```python
from build123d import *

# Parameters (mm, degrees)
BOSS_EXTRUDE1_DEPTH = 80
SKETCH2_R           = 21.75
CUT_EXTRUDE1_DEPTH  = 10
SKETCH3_R           = 1.4
CUT_EXTRUDE2_DEPTH  = 4
CUT_EXTRUDE3_DEPTH  = 6
SKETCH5_R           = 2.25
CUT_EXTRUDE4_DEPTH  = 81
SKETCH6_W           = 10.75
SKETCH6_H           = 28.5
CUT_EXTRUDE5_DEPTH  = 28.5
BOSS_EXTRUDE2_DEPTH = 100
SKETCH8_W           = 5
SKETCH8_H           = 28.5
CUT_EXTRUDE6_DEPTH  = 80
SKETCH9_R           = 24
CUT_EXTRUDE7_DEPTH  = 80
SKETCH12_R          = 6
CUT_EXTRUDE9_DEPTH  = 28
SKETCH13_W          = 58.5
SKETCH13_H          = 5
CUT_EXTRUDE10_DEPTH = 28.5
FILLET2_R           = 2
SKETCH15_R          = 1.5
CUT_EXTRUDE11_DEPTH = 28.5


with BuildPart() as part:
    # Sketch1 → Boss-Extrude1 (new body)
    with BuildSketch(Plane(origin=(0, 0, 0), x_dir=(1, 0, 0), z_dir=(0, 1, 0))):
        Polygon((-40, -13.75), (40, -13.75), (40, 13.75), (29.25, 13.75), (29.25, -3.75), (-29.25, -3.75), (-29.25, 13.75), (-40, 13.75), align=None)
    extrude(amount=BOSS_EXTRUDE1_DEPTH)

    # Sketch2 → Cut-Extrude1 (cut)
    with BuildSketch(Plane.XY.offset(13.75)):
        with Locations((0, 35.5)):
            Circle(SKETCH2_R)
    extrude(amount=-CUT_EXTRUDE1_DEPTH, mode=Mode.SUBTRACT)

    # Sketch3 → Cut-Extrude2 (cut)
    with BuildSketch(Plane.XY.offset(13.75)):
        with Locations((26, 65)):
            Circle(SKETCH3_R)
        with Locations((-26, 65)):
            Circle(SKETCH3_R)
    extrude(amount=-CUT_EXTRUDE2_DEPTH, mode=Mode.SUBTRACT)

    # Sketch4 → Cut-Extrude3 (cut)
    with BuildSketch(Plane(origin=(0, 0, 3.75), x_dir=(-1, 0, 0), z_dir=(0, 0, -1))):
        Polygon((-27.21, 62.904218523), (-28.42, 65), (-27.21, 67.095781477), (-24.79, 67.095781477), (-23.58, 65), (-24.79, 62.904218523), align=None)
        Polygon((28.42, 65), (27.21, 67.095781477), (24.79, 67.095781477), (23.58, 65), (24.79, 62.904218523), (27.21, 62.904218523), align=None)
    extrude(amount=-CUT_EXTRUDE3_DEPTH, mode=Mode.SUBTRACT)

    # Sketch5 → Cut-Extrude4 (cut, through all)
    with BuildSketch(Plane(origin=(40, 0, 0), x_dir=(0, 0, -1), z_dir=(1, 0, 0))):
        with Locations((5.75, 18.5)):
            Circle(SKETCH5_R)
        with Locations((5.75, 37)):
            Circle(SKETCH5_R)
    extrude(amount=-CUT_EXTRUDE4_DEPTH, mode=Mode.SUBTRACT)

    # Sketch6 → Cut-Extrude5 (cut, through all)
    with BuildSketch(Plane.XY.offset(13.75)):
        with Locations((-34.625, 65.75)):
            Rectangle(SKETCH6_W, SKETCH6_H)
        with Locations((34.625, 65.75)):
            Rectangle(SKETCH6_W, SKETCH6_H)
    extrude(amount=-CUT_EXTRUDE5_DEPTH, mode=Mode.SUBTRACT)

    # Sketch7 → Boss-Extrude2 (add)
    with BuildSketch(Plane.ZY.offset(40)):
        Polygon((3.75, 0), (3.75, -22), (13.75, -22), (13.75, 0), (13.75, 80), (3.75, 80), align=None)
    extrude(amount=BOSS_EXTRUDE2_DEPTH)

    # Sketch8 → Cut-Extrude6 (cut)
    with BuildSketch(Plane.XY.offset(13.75)):
        with Locations((-42.5, 65.75)):
            Rectangle(SKETCH8_W, SKETCH8_H)
        with Locations((-137.5, 65.75)):
            Rectangle(SKETCH8_W, SKETCH8_H)
    extrude(amount=-CUT_EXTRUDE6_DEPTH, mode=Mode.SUBTRACT)

    # Sketch9 → Cut-Extrude7 (cut)
    with BuildSketch(Plane.XY.offset(13.75)):
        with Locations((-108, 7.5)):
            Circle(SKETCH9_R)
    extrude(amount=-CUT_EXTRUDE7_DEPTH, mode=Mode.SUBTRACT)

    # Sketch12 → Cut-Extrude9 (cut)
    with BuildSketch(Plane.XY.offset(13.75)):
        with Locations((-70, 52)):
            Circle(SKETCH12_R)
    extrude(amount=-CUT_EXTRUDE9_DEPTH, mode=Mode.SUBTRACT)

    # Sketch13 → Cut-Extrude10 (cut, through all)
    with BuildSketch(Plane.XY.offset(13.75)):
        with Locations((0, 77.5)):
            Rectangle(SKETCH13_W, SKETCH13_H)
    extrude(amount=-CUT_EXTRUDE10_DEPTH, mode=Mode.SUBTRACT)

    # Fillet2
    fillet2_edges = [part.edges().sort_by_distance(p)[0] for p in [
        (-29.25, 51.5, 8.75),
        (29.25, 51.5, 8.75),
        (40, 51.5, 0),
        (-40, 0, 8.75),
        (-40, -22, 8.75),
        (-140, -22, 8.75),
        (-140, 51.5, 8.75),
        (-45, 51.5, 8.75),
        (-45, 80, 8.75),
        (-135, 80, 8.75),
        (-135, 51.5, 8.75),
        (-29.25, 75, 8.75),
        (29.25, 75, 8.75),
        (40, 0, 0),
    ]]
    fillet(fillet2_edges, radius=FILLET2_R)

    # Sketch15 → Cut-Extrude11 (cut, through all)
    with BuildSketch(Plane.XY.offset(13.75)):
        with Locations((-57.272077939, 64.727922061)):
            Circle(SKETCH15_R)
        with Locations((-57.272077939, 39.272077939)):
            Circle(SKETCH15_R)
        with Locations((-82.727922061, 39.272077939)):
            Circle(SKETCH15_R)
        with Locations((-82.727922061, 64.727922061)):
            Circle(SKETCH15_R)
    extrude(amount=-CUT_EXTRUDE11_DEPTH, mode=Mode.SUBTRACT)


solid = part.part
```
Design review of the part built by this model. Coordinates are the model's own, in mm. A direction names the side the tool comes from. Coordinates: 2 decimals unless noted, no trailing zeros. Loops run counter-clockwise (first coordinate to the right, second up) from the corner with the lowest first, then second, coordinate; pieces in that order, holes last. Notation, with made-up numbers: M -34,87.25 L 3,87.25 A9 ccw 3,91.25 Z; hole C 47.25,15 d6. An arc over 180 degrees is marked long. One line per question, with ' | ' between items.
(1) Machinability: for faces 1 (the face through (29.25, 63, 9)), 2 (the face through (-40, -11, 9)), 3 (the face through (-40, 25, -5)), which of the approach directions +Z, -Z, +X, -X, +Y, -Y give a long, thin tool a straight path to every point of the face, cutting with its end or side? Answer none if there is none.
Filled in:
face 1: +Z, -Z, +X, +Y | face 2: +Z, -Z, +X, -Y | face 3: -Z, -X, +Y, -Y
(2) For pin 1 Ø2.5 at (x, z) = (-25.5, 5.5) entering from -Y; pin 2 Ø5 at (y, z) = (-10.5, 10.5) entering from +X; pin 3 Ø19 at (x, y) = (-70, 52) entering from -Z; pin 4 Ø12 at (x, y) = (-28, 22.5) entering from -Z, all flat-tipped, find the tip position at first contact; note any pin that passes through.
Filled in:
pin 1: stops at y = 0 | pin 2: stops at x = -40 | pin 3: stops at z = 3.75 | pin 4: stops at z = -13.75
(3) We need section A-A (x = -70). Give the boundary of the cut face in (y, z), and give its area (3 significant figures).
Filled in:
outline: M -22,3.75 L 46,3.75 L 46,13.75 L -22,13.75 Z; M 58,3.75 L 80,3.75 L 80,13.75 L 58,13.75 Z | area: 900 mm^2
(4) We need section B-B (z = -5.75). Give the boundary of the cut face in (x, y), and give its area (3 significant figures).
Filled in:
outline: M -40,0 L -29.25,0 L -29.25,16.25 L -40,16.25 Z; M -40,20.75 L -29.25,20.75 L -29.25,34.75 L -40,34.75 Z; M -40,39.25 L -29.25,39.25 L -29.25,51.5 L -40,51.5 Z; M 29.25,0 L 38,0 A2 ccw 40,2 L 40,16.25 L 29.25,16.25 Z; M 29.25,20.75 L 40,20.75 L 40,34.75 L 29.25,34.75 Z; M 29.25,39.25 L 40,39.25 L 40,49.5 A2 ccw 38,51.5 L 29.25,51.5 Z | area: 912 mm^2
(5) Draft analysis for pull direction Y (two halves, no side actions). For faces 4 (the face through (-45, 66, 9)), 5 (the face through (-131.977, 8.555, 8.82)), 6 (the face through (-2, 0, 6)), state which applies: released by +Y, released by -Y, zero draft, split by the parting line, or undercut.
Filled in:
face 4: zero draft | face 5: undercut | face 6: released by -Y
(6) We need section C-C (y = 60). Give the boundary of the cut face in (x, z).
Filled in:
outline: M -135,3.75 L -45,3.75 L -45,13.75 L -135,13.75 Z; M -29.25,3.75 L 29.25,3.75 L 29.25,13.75 L -29.25,13.75 Z
(7) Wall thickness on probe 1 along Y at (x, z) = (26, 11.1); probe 2 along Y at (x, z) = (35.25, -5.75); probe 3 along X at (y, z) = (39.5, 12.5): over which ranges is each line inside the solid? List them lowest first.
Filled in:
probe 1: y = 0 to 63.6, 66.4 to 75 | probe 2: y = 0 to 16.25, 20.75 to 34.75, 39.25 to 51.5 | probe 3: x = -140 to -84.21, -81.25 to -58.75, -55.79 to -21.38, 21.38 to 40
(8) We need section D-D (y = 23). Give the boundary of the cut face in (x, z), and give its area (3 significant figures).
Filled in:
outline: M -140,3.75 L -126.32,3.75 L -126.32,13.75 L -140,13.75 Z; M -89.68,3.75 L -40,3.75 L -40,-13.75 L -29.25,-13.75 L -29.25,3.75 L -17.8,3.75 L -17.8,13.75 L -89.68,13.75 Z; M 17.8,3.75 L 29.25,3.75 L 29.25,-13.75 L 40,-13.75 L 40,13.75 L 17.8,13.75 Z | area: 1,450 mm^2
